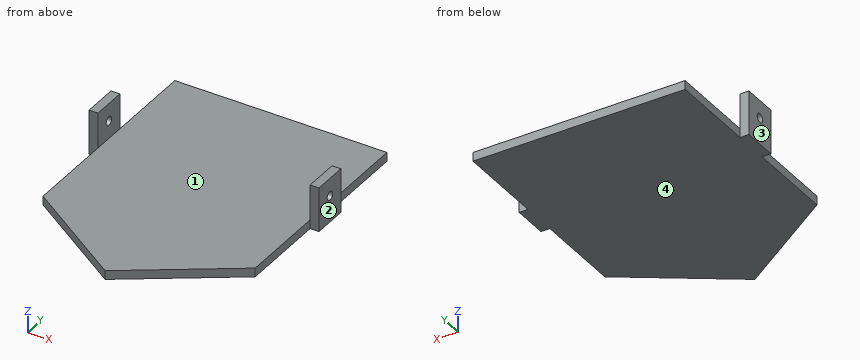
from build123d import *

# Parameters (mm, degrees)
F1_DEPTH  = 3.175
F2_W      = 12.7
F2_H      = 12.7
F2_R      = 1.5875
F4_DEPTH  = 3.175
F4_FACE_W = 3.175
F4_FACE_H = 12.7
F5_DEPTH  = 3.175
F3_W      = 12.7
F3_H      = 12.7
F3_R      = 1.5875
F6_DEPTH  = 3.175
F6_FACE_W = 3.175
F6_FACE_H = 12.7
F7_DEPTH  = 3.175


with BuildPart() as f1:
    # F0 (on Top) → F1 (new body)
    with BuildSketch(Plane.XY):
        Polygon((29.825334, 66.574713), (-46.374666, 66.574713), (-46.374666, -9.625287), (-8.274666, -35.025287), (29.825334, -9.625287), align=None)
    extrude(amount=F1_DEPTH)



with BuildPart() as f4:
    # F2 (on face) → F4 (new body)
    with BuildSketch(Plane(origin=(-46.374666, 0, 0), x_dir=(0, -1, 0), z_dir=(-1, 0, 0))):
        with Locations((-28.474713, 9.525)):
            Rectangle(F2_W, F2_H)
        with Locations((-28.474713, 9.525)):
            Circle(F2_R, mode=Mode.SUBTRACT)
    extrude(amount=F4_DEPTH)


with BuildPart() as f1_1:
    add(f1.part)

    add(f4.part)  # F5 merges F4
    # F4_face (on face) → F5 (join)
    with BuildSketch(Plane(origin=(-47.962166, 28.474713, 3.175), x_dir=(1, 0, 0), z_dir=(0, 0, -1))):
        Rectangle(F4_FACE_W, F4_FACE_H)
    extrude(amount=F5_DEPTH)



with BuildPart() as f6:
    # F3 (on face) → F6 (new body)
    with BuildSketch(Plane.YZ.offset(29.825334)):
        with Locations((28.474713, 9.525)):
            Rectangle(F3_W, F3_H)
        with Locations((28.474713, 9.525)):
            Circle(F3_R, mode=Mode.SUBTRACT)
    extrude(amount=F6_DEPTH)


with BuildPart() as f1_2:
    add(f1_1.part)

    add(f6.part)  # F7 merges F6
    # F6_face (on face) → F7 (join)
    with BuildSketch(Plane(origin=(31.412834, 28.474713, 3.175), x_dir=(1, 0, 0), z_dir=(0, 0, -1))):
        Rectangle(F6_FACE_W, F6_FACE_H)
    extrude(amount=F7_DEPTH)


solid = f1_2.part
For this review, take the finished solid that the model builds, in its own axes (mm). Face numbers are marked on the shaded views. Round coordinates to 2 decimals unless told otherwise and drop trailing zeros. Write each loop counter-clockwise with the first axis right and the second up, starting at its lowest first coordinate (ties: lowest second). Pieces come first, ordered by that corner, then holes. Notation, with made-up numbers: (24.25, -15) -> (33.25, -15) arc R18 cw to (33.25, 20) -> close; hole circle Ø9 at (-35, 21). An arc over 180 degrees is marked (long way). Use CSV: the item, a comma, the result in double quotes.
(1) Draft analysis for pull direction X (two halves, no side actions). For the marked faces 1, 2, 3 and 4, state which applies: +X half, -X half, draft (parallel to the pull), parting line (faces both ways), or undercut.
Computed values:
face 1,"undercut"
face 2,"+X half"
face 3,"-X half"
face 4,"draft"
(2) Consider section B-B, the plane y = 28.5. Give the boundary of the cut face in (x, z) (3 decimals).
Computed values:
outline,"(-49.55, 0) -> (33, 0) -> (33, 7.938) -> (29.825, 7.938) -> (29.825, 3.175) -> (-46.375, 3.175) -> (-46.375, 7.938) -> (-49.55, 7.938) -> close; (-49.55, 11.112) -> (-46.375, 11.112) -> (-46.375, 15.875) -> (-49.55, 15.875) -> close; (29.825, 11.112) -> (33, 11.112) -> (33, 15.875) -> (29.825, 15.875) -> close"
(3) Consider section C-C, the plane z = 1.25. Give the boundary of the cut face in (x, y).
Computed values:
outline,"(-49.55, 22.12) -> (-46.37, 22.12) -> (-46.37, -9.63) -> (-8.27, -35.03) -> (29.83, -9.63) -> (29.83, 22.12) -> (33, 22.12) -> (33, 34.82) -> (29.83, 34.82) -> (29.83, 66.57) -> (-46.37, 66.57) -> (-46.37, 34.82) -> (-49.55, 34.82) -> close"
(4) Consider section D-D, the plane y = 5. Give the boundary of the cut face in (x, z) (3 decimals).
Computed values:
outline,"(-46.375, 0) -> (29.825, 0) -> (29.825, 3.175) -> (-46.375, 3.175) -> close"
(5) To check wall thickness, follow L1, parallel to Z at x = 14, y = -13 (3 decimals); L2, parallel to X at y = 24, z = 10.5; L3, parallel to Y at x = 22.5, z = 3. State the ranges of each line that lie inside material, in increasing order. Write a range as [from, to].
Computed values:
L1,"[0, 3.175]"
L2,"[-49.55, -46.37], [29.83, 33]"
L3,"[-14.51, 66.57]"
(6) Clearance check with flat-ended pins moving along their axes: P1, Ø23, axis at x = -15.5, y = 0, coming from the +Z side (3 decimals); P2, Ø3.5, axis at x = 31, z = 7, coming from the -Y side; P3, Ø2.5, axis at y = 8, z = 1.5, coming from the -X side; P4, Ø3, axis at y = 28.47, z = 9.52, coming from the -X side. State where each tip first meets the part, or that it passes through.
Computed values:
P1,"z = 3.175"
P2,"y = 22.12"
P3,"x = -46.37"
P4,"through"
(7) Consider section A-A, the plane z = 13.75. Give the boundary of the cut face in (x, y).
Computed values:
outline,"(-49.55, 22.12) -> (-46.37, 22.12) -> (-46.37, 34.82) -> (-49.55, 34.82) -> close; (29.83, 22.12) -> (33, 22.12) -> (33, 34.82) -> (29.83, 34.82) -> close"
